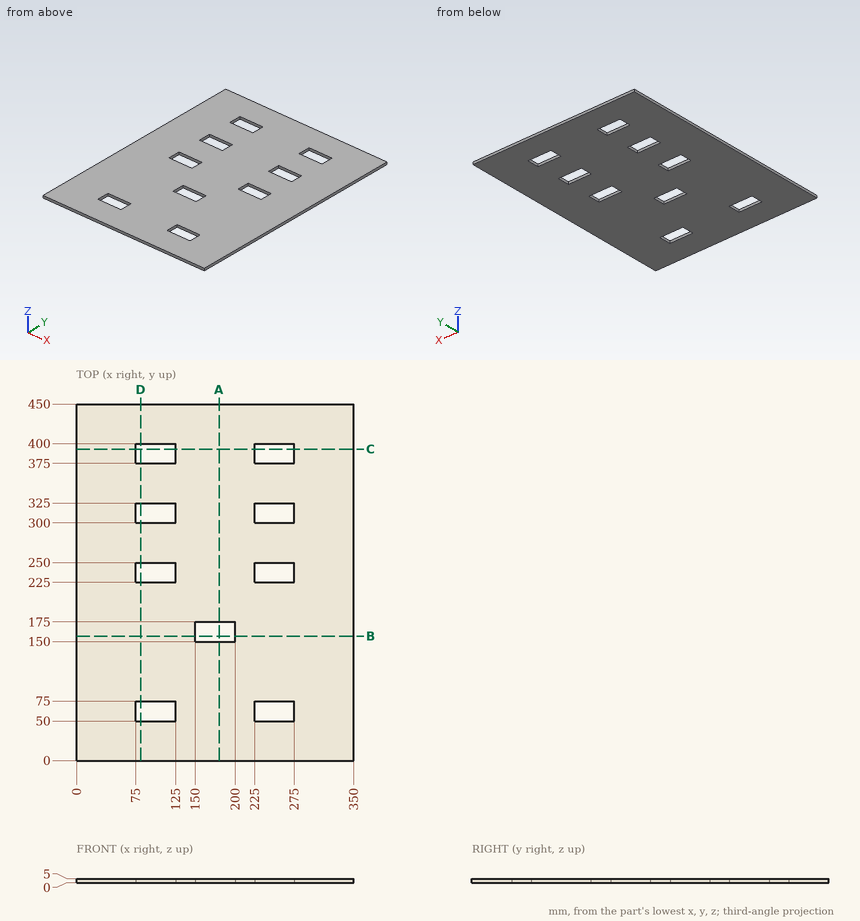
Drawing for the job (mm, zero at the part's lowest x, y, z). Coordinates: 2 decimals unless noted, no trailing zeros. Loops run counter-clockwise (first coordinate to the right, second up) from the corner with the lowest first, then second, coordinate; pieces in that order, holes last. Notation, with made-up numbers: (65, 50) - (117, 50) arc R24 ccw to (117, 78) - close; hole circle Ø8 at (35.5, 71.5). An arc over 180 degrees is marked (long way). Use CSV: the item, a comma, the result in double quotes. Start each with the question number.
Q1. Cut at A-A, the plane x = 180. List the corners of the cut face in (y, z).
Q2. Cut at B-B, the plane y = 157. List the corners of the cut face in (x, z).
Q3. Cut at C-C, the plane y = 393. List the corners of the cut face in (x, z), then the cut area to 3 significant figures.
Q4. Probe probe 1 along Y at (x, z) = (80, 4.6); probe 2 along X at (y, z) = (66.5, 1.2); probe 3 along X at (y, z) = (150.5, 4.35). List the from-to ranges inside material, lowest first. Write a range as from..to.
Q5. Cut at D-D, the plane x = 81. List the corners of the cut face in (y, z), then the cut area to 3 significant figures.
Here are the results:
1,outline,"(0, 0) - (150, 0) - (150, 5) - (0, 5) - close; (175, 0) - (450, 0) - (450, 5) - (175, 5) - close"
2,outline,"(0, 0) - (150, 0) - (150, 5) - (0, 5) - close; (200, 0) - (350, 0) - (350, 5) - (200, 5) - close"
3,outline,"(0, 0) - (75, 0) - (75, 5) - (0, 5) - close; (125, 0) - (225, 0) - (225, 5) - (125, 5) - close; (275, 0) - (350, 0) - (350, 5) - (275, 5) - close"
3,area,"1,250 mm2"
4,probe 1,"0..50, 75..225, 250..300, 325..375, 400..450"
4,probe 2,"0..75, 125..225, 275..350"
4,probe 3,"0..150, 200..350"
5,outline,"(0, 0) - (50, 0) - (50, 5) - (0, 5) - close; (75, 0) - (225, 0) - (225, 5) - (75, 5) - close; (250, 0) - (300, 0) - (300, 5) - (250, 5) - close; (325, 0) - (375, 0) - (375, 5) - (325, 5) - close; (400, 0) - (450, 0) - (450, 5) - (400, 5) - close"
5,area,"1,750 mm2"
